Design review of the part built by this model. Coordinates are the model's own, in mm. Face numbers are marked on the shaded views. A direction names the side the tool comes from. Coordinates: 2 decimals unless noted, no trailing zeros. Order: outer loops, then holes, each group sorted by start corner. A loop starts at its lowest first (then second) coordinate and runs counter-clockwise, first axis right, second up. Notation, with made-up numbers: M 85.5,-35 L 102.5,-35 A23 ccw 102.5,-25 Z; hole C 51.5,29.25 d10. An arc over 180 degrees is marked long. Use CSV: the item, a comma, the result in double quotes.
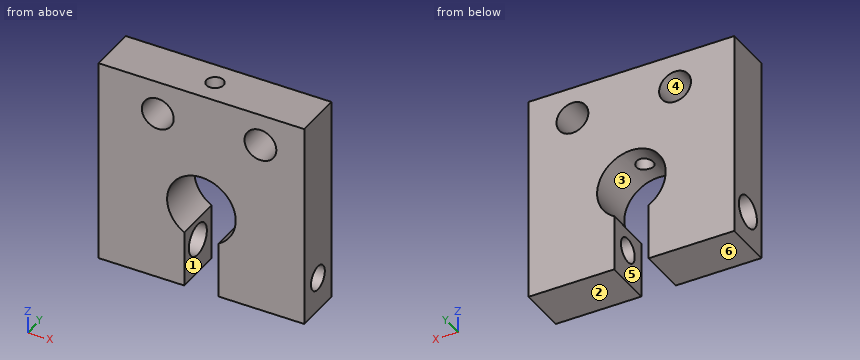
```python
from build123d import *

# Parameters (mm, degrees)
SKETCH1_W           = 19.05
SKETCH1_H           = 19.05
SKETCH1_R           = 3.175
BOSS_EXTRUDE1_DEPTH = 4.445
SKETCH2_R           = 1.4732
SKETCH2_W           = 3.175
SKETCH2_H           = 5.187869343
CUT_EXTRUDE1_DEPTH  = 16.296120627
SKETCH4_R           = 0.7874
CUT_EXTRUDE3_DEPTH  = 22.757438958
SKETCH6_R           = 1.1303
CUT_EXTRUDE5_DEPTH  = 16.296120729
SKETCH7_R           = 1.4732
CUT_EXTRUDE6_DEPTH  = 16.296120729


with BuildPart() as part:
    # Sketch1 → Boss-Extrude1 (new body)
    with BuildSketch(Plane(origin=(0, 0, 0), x_dir=(1, 0, 0), z_dir=(0, 1, 0))):
        with Locations((0, -1.5875)):
            Rectangle(SKETCH1_W, SKETCH1_H)
        with Locations(Location((0, 0, 0), (0, 0, 270))):
            Circle(SKETCH1_R, mode=Mode.SUBTRACT)
    extrude(amount=BOSS_EXTRUDE1_DEPTH)

    # Sketch2 → Cut-Extrude1 (cut, through all)
    with BuildSketch(Plane(origin=(0, 4.445, 0), x_dir=(1, 0, 0), z_dir=(0, 1, 0))):
        with Locations(Location((5.461, -8.1788, 0), (0, 0, 270))):
            Circle(SKETCH2_R)
        with Locations(Location((-4.0386, -8.0264, 0), (0, 0, 270))):
            Circle(SKETCH2_R)
        with Locations((0, 5.343565329)):
            Rectangle(SKETCH2_W, SKETCH2_H)
    extrude(amount=-CUT_EXTRUDE1_DEPTH, mode=Mode.SUBTRACT)

    # Sketch4 → Cut-Extrude3 (cut, through all)
    with BuildSketch(Plane.XY.offset(11.1125)):
        with Locations((0, 2.2225)):
            Circle(SKETCH4_R)
    extrude(amount=-CUT_EXTRUDE3_DEPTH, mode=Mode.SUBTRACT)

    # Sketch6 → Cut-Extrude5 (cut, through all)
    with BuildSketch(Plane(origin=(0, 0, 0), x_dir=(0, 0, -1), z_dir=(1, 0, 0))):
        with Locations(Location((4.7625, 2.2225, 0), (0, 0, 180))):
            Circle(SKETCH6_R)
    extrude(amount=CUT_EXTRUDE5_DEPTH, mode=Mode.SUBTRACT)

    # Sketch7 → Cut-Extrude6 (cut, through all)
    with BuildSketch(Plane(origin=(0, 0, 0), x_dir=(0, 0, -1), z_dir=(1, 0, 0))):
        with Locations((4.7625, 2.2225)):
            Circle(SKETCH7_R)
    extrude(amount=-CUT_EXTRUDE6_DEPTH, mode=Mode.SUBTRACT)


solid = part.part
```
(1) Wall thickness on probe 1 along X at (y, z) = (3.6, -4) (1 decimal); probe 2 along X at (y, z) = (3, 0) (3 decimals); probe 3 along Z at (x, y) = (-5, 1.5): over which ranges is each line inside the solid? List them lowest first.
The answers:
probe 1,"x = -9.5 to -1.6, 1.6 to 9.5"
probe 2,"x = -9.525 to -3.175, 3.175 to 9.525"
probe 3,"z = -7.94 to -6.05, -3.48 to 6.91, 9.14 to 11.11"
(2) Add section D-D on x = 0. State the section outline as (y, z) points (1 decimal).
The answers:
outline,"M 0,3.2 L 1.4,3.2 L 1.4,11.1 L 0,11.1 Z; M 3,3.2 L 4.4,3.2 L 4.4,11.1 L 3,11.1 Z"
(3) Add section B-B on z = 0. State the section outline as (x, y) points (3 decimals), and give its area (3 significant figures).
The answers:
outline,"M -9.525,0 L -3.175,0 L -3.175,4.445 L -9.525,4.445 Z; M 3.175,0 L 9.525,0 L 9.525,4.445 L 3.175,4.445 Z"
area,"56.5 mm2"
(4) Add section A-A on z = 9.25. State the section outline as (x, y) points (1 decimal), and give its area (3 significant figures).
The answers:
outline,"M -9.5,0 L -4.9,0 L -4.9,4.4 L -9.5,4.4 Z; M -3.2,0 L 4.4,0 L 4.4,4.4 L -3.2,4.4 Z; M 6.5,0 L 9.5,0 L 9.5,4.4 L 6.5,4.4 Z; hole C 0,2.2 d1.6"
area,"66.4 mm2"
(5) The part is to be moulded in two halves that separate along Z. For the marked faces 1, 2, 3 and 4, say which applies: pulls with the +Z half, pulls with the -Z half, needs draft (parallel to the pull), parting line crosses it, or undercut.
The answers:
face 1,"needs draft"
face 2,"pulls with the -Z half"
face 3,"undercut"
face 4,"undercut"
(6) Add section C-C on y = 1.75. Give the number of separate pieces and of enclosed holes in the cut face, and give its area (3 significant figures).
The answers:
separate pieces,"4"
enclosed holes,"2"
area,"254 mm2"
(7) Clearance check with a flat-ended pin moving along its axis: P1, Ø2.5, axis at x = 0, y = 2.22, coming from the -Z side. State where the tip first meets the part, or that it passes through.
The answers:
P1,"stops at z = 2.92"
(8) For the marked faces 5 and 6, list the 3-axis set-ups (+Z, -Z, +X, -X, +Y, -Y) from which the entire face can be reached by the end or side of a thin tool; tool diameter is ignored.
The answers:
face 5,"-Z, +Y, -Y"
face 6,"-Z, +X, -X, +Y, -Y"
